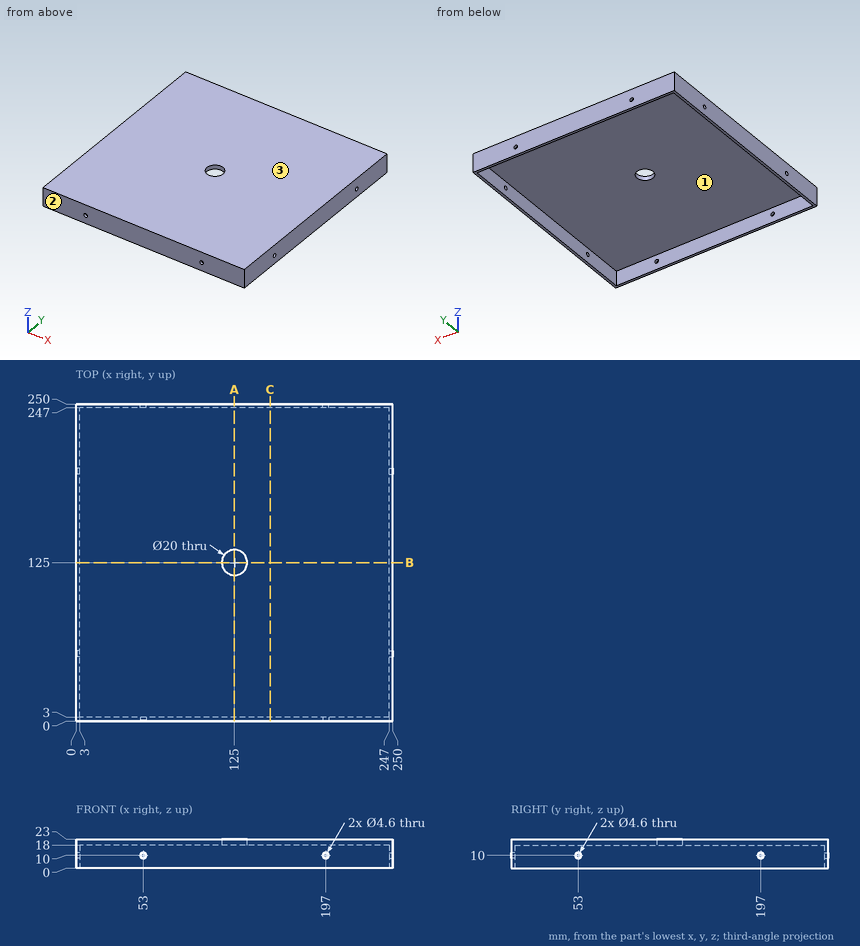
Design review of the part shown in the three views and the two pictorial views. Dimensions are in mm from the part's minimum x, y and z. Give positions to 0.01 mm unless a question says otherwise; leave off trailing zeros. Order: outer loops, then holes, each group sorted by start corner. A loop starts at its lowest first (then second) coordinate and runs counter-clockwise, first axis right, second up. Notation, with made-up numbers: M 45,76 L 71,76 A6 cw 71,80 Z; hole C -24,-22 d6. An arc over 180 degrees is marked long. Answer in a Markdown table with one row per item. Add a question column.
(1) For pin 1 (5.5 mm diameter, centred on y = 53, z = 10, fed in from +X); pin 2 (6 mm diameter, centred on x = 99, y = 35.5, fed in from -Z), all flat-tipped, find the tip position at first contact; note any pin that passes through.
(2) Mouldability with a two-part tool opening along Y and no side actions: class the marked faces 1, 2 and 3 as +Y half, -Y half, draft (parallel to the pull), parting line (faces both ways), or undercut.
(3) Wall thickness on probe 1 along Y at (x, z) = (1.25, 10); probe 2 along X at (y, z) = (93, 7): over which ranges is each line inside the solid? List them lowest first. Write a range as [from, to].
(4) Consider section C-C on x = 153. State the section outline as (y, z) points.
(5) Consider section A-A on x = 125. State the section outline as (y, z) points.
Evaluation:
| question | item | result |
|---|---|---|
| 1 | pin 1 | stops at x = 250 |
| 1 | pin 2 | stops at z = 18 |
| 2 | face 1 | undercut |
| 2 | face 2 | -Y half |
| 2 | face 3 | draft |
| 3 | probe 1 | y = [0, 50.7], [55.3, 194.7], [199.3, 250] |
| 3 | probe 2 | x = [0, 3], [247, 250] |
| 4 | outline | M 0,0 L 3,0 L 3,18 L 247,18 L 247,0 L 250,0 L 250,23 L 0,23 Z |
| 5 | outline | M 0,0 L 3,0 L 3,18 L 115,18 L 115,23 L 0,23 Z; M 135,18 L 247,18 L 247,0 L 250,0 L 250,23 L 135,23 Z |
